Model file for the job. Use its own axes, mm. A direction names the side the tool comes from. Give positions to 0.01 mm unless a question says otherwise; leave off trailing zeros. Order: outer loops, then holes, each group sorted by start corner. A loop starts at its lowest first (then second) coordinate and runs counter-clockwise, first axis right, second up. Notation, with made-up numbers: (84, 33) - (91, 33) arc R8 cw to (91, 45) - close; hole circle Ø2 at (35.25, -1.75). An arc over 180 degrees is marked (long way). Use CSV: the item, a comma, the result in double quotes. Start each with the question number.
(1) Tool access for faces 4 (the flat face through (915, 1029, -57.15)), 5 (the flat face through (964, 1365, 28.575)), 6 (the flat face through (464, 2057.4, -29)), 7 (the flat face through (-15.875, 1038, 22)): list every direction of +Z, -Z, +X, -X, +Y, -Y with a clear straight run to the whole face (end or side of a thin tool).
(2) Pull direction X, two halves, no side cores. Call faces 1 (the flat face through (-25.4, 1043, -29)), 2 (the flat face through (464, 2032, -28)), 3 (the flat face through (938, 0, -28)): +X half, -X half, draft (parallel to the pull), parting line (faces both ways), or undercut.
(3) Band-saw the part on C-C, the plane z = -27.5. Give the cut face in (x, y), then the cut area to 3 significant figures.
(4) Drop flat-ended pins along their axis: pin 1 Ø10 at (x, z) = (600, -46.5) entering from -Y; pin 2 Ø1 at (x, z) = (537, -4.5) entering from +Y; pin 3 Ø1 at (y, z) = (1144, -1.5) entering from -X. Give the stop position or say it passes through.
(5) Probe L1, parallel to X at y = 526, z = 19 (3 decimals); L2, parallel to X at y = 780, z = -33.5; L3, parallel to Y at x = 705.5, z = 33.5 (3 decimals). List the from-to ranges inside material, lowest first.
from build123d import *


with BuildPart() as part:
    # Sweep1: sweep along a path in Sketch1
    with BuildLine(Plane.XY) as sweep1_path:
        Line((0, 0), (0, 2032))
        Line((0, 2032), (914.4, 2032))
        Line((914.4, 2032), (914.4, 0))
    # Sketch2 → Sweep1 (sweep)
    with BuildSketch(Plane(origin=(0, 0, 0), x_dir=(1, 0, 0), z_dir=(0, 1, 0))):
        Polygon((0, 0), (0, 57.15), (-15.875, 57.15), (-15.875, 100.0125), (-66.675, 100.0125), (-66.675, 85.725), (-25.4, 85.725), (-25.4, -28.575), (-66.675, -28.575), (-66.675, -42.8625), (-15.875, -42.8625), (-15.875, 0), align=None)
    sweep(path=sweep1_path.line, transition=Transition.RIGHT)


solid = part.part
Answer block:
1,face 4,"-Z, -Y"
1,face 5,"+Y"
1,face 6,"+X, -X, +Y"
1,face 7,"+Z, -Y"
2,face 1,"-X half"
2,face 2,"undercut"
2,face 3,"draft"
3,outline,"(-25.4, 0) - (0, 0) - (0, 2032) - (914.4, 2032) - (914.4, 0) - (939.8, 0) - (939.8, 2057.4) - (-25.4, 2057.4) - close"
3,area,"128,000 mm2"
4,pin 1,"stops at y = 2032"
4,pin 2,"stops at y = 2057.4"
4,pin 3,"stops at x = -25.4"
5,L1,"x = -25.4 to -15.875, 930.275 to 939.8"
5,L2,"x = -25.4 to 0, 914.4 to 939.8"
5,L3,"y = 2047.875 to 2098.675"
